Read the model definition and answer for the solid it produces. Units are mm, in the model's axes. A direction names the side the tool comes from. Give positions to 0.01 mm unless a question says otherwise; leave off trailing zeros. Order: outer loops, then holes, each group sorted by start corner. A loop starts at its lowest first (then second) coordinate and runs counter-clockwise, first axis right, second up. Notation, with made-up numbers: (-17.5, -27.5) - (19.5, -27.5) arc R38 cw to (19.5, 10.5) - close; hole circle Ø5 at (14.25, -26). An arc over 180 degrees is marked (long way). Use a Markdown table: item, result. Add a question column.
1. Which of the six approach directions +Z, -Z, +X, -X, +Y, -Y give full straight-line access (tool end or side, diameter ignored) to faces 3 (the flat face through (-1, 7, 0)), 4 (the flat face through (117, 5, -2)), 5 (the flat face through (-1, 3, 30))?
2. A cutting plane is placed at C-C on x = 26.5. Determine the outline of the cut face in (y, z), and give its area (3 significant figures).
3. Consider L1, parallel to X at y = 2.55, z = 90; L2, parallel to X at y = 1, z = 115; L3, parallel to X at y = 4.5, z = 99.5. Determine where each line is inside the solid, lowest interval first.
4. Flat-ended cylindrical pins translate along their axes: P1, Ø6.5, axis at x = -130, z = 115, coming from the -Y side; P2, Ø3, axis at x = -90, y = 1, coming from the -Z side; P3, Ø4.5, axis at x = -129, z = 70, coming from the +Y side; P4, Ø4, axis at x = -92, y = 3.5, coming from the +Z side. Find the tip coordinate at first contact, or state that the pin passes through.
5. A cutting plane is placed at A-A on z = -51.5. Determine the outline of the cut face in (x, y).
6. A cutting plane is placed at B-B on y = 1.25. State how many separate pieces and enclosed holes the cut face has, and give its area (3 significant figures).
7. For a pull along X with two mould halves and no side action, classify faces 1 (the flat face through (-1, 3, -30)), 2 (the flat face through (-118, 5, -2)) as released by +X, released by -X, zero draft, split by the parting line, or undercut.
```python
from build123d import *

# Parameters (mm, degrees)
SKETCH1_W             = 45
SKETCH1_H             = 250
BOSS_EXTRUDE1_DEPTH   = 5
BOSS_EXTRUDE1_2_DEPTH = 5
SKETCH2_W             = 190
SKETCH2_H             = 60
BOSS_EXTRUDE2_DEPTH   = 7
CHAMFER1_SIZE         = 2
FILLET1_R             = 2
SKETCH3_R             = 2
CUT_EXTRUDE1_DEPTH    = 188.749833555
LPATTERN1_COUNT       = 2
LPATTERN1_PITCH       = 240
LPATTERN1_COUNT_DIR2  = 2
LPATTERN1_PITCH_DIR2  = 160
SKETCH4_R             = 4
CUT_EXTRUDE2_DEPTH    = 188.749833555
LPATTERN2_COUNT       = 2
LPATTERN2_PITCH       = 260
LPATTERN2_COUNT_DIR2  = 2
LPATTERN2_PITCH_DIR2  = 230


with BuildPart() as part:
    # Sketch1 → Boss-Extrude1 (new body)
    with BuildSketch(Plane(origin=(0, 0, 0), x_dir=(1, 0, 0), z_dir=(0, 1, 0))):
        with Locations((-117.5, 0)):
            Rectangle(SKETCH1_W, SKETCH1_H)
    extrude(amount=BOSS_EXTRUDE1_DEPTH)



with BuildPart() as body_2:
    # Sketch1 → Boss-Extrude1 2 (new body)
    with BuildSketch(Plane(origin=(0, 0, 0), x_dir=(1, 0, 0), z_dir=(0, 1, 0))):
        with Locations((117.5, 0)):
            Rectangle(SKETCH1_W, SKETCH1_H)
    extrude(amount=BOSS_EXTRUDE1_2_DEPTH)


with BuildPart() as part_1:
    add(part.part)

    add(body_2.part)  # Boss-Extrude2 merges body 2
    # Sketch2 → Boss-Extrude2 (add)
    with BuildSketch(Plane(origin=(0, 0, 0), x_dir=(1, 0, 0), z_dir=(0, 1, 0))):
        Rectangle(SKETCH2_W, SKETCH2_H)
    extrude(amount=BOSS_EXTRUDE2_DEPTH)

    # Chamfer1
    chamfer1_edges = [part_1.edges().sort_by_distance(p)[0] for p in [
        (95, 7, 0),
        (-95, 7, 0),
    ]]
    chamfer(chamfer1_edges, length=CHAMFER1_SIZE - 0.0001)  # a hair under: the kernel refuses the full size

    # Fillet1
    fillet1_edges = [part_1.edges().sort_by_distance(p)[0] for p in [
        (95, 2.5, -125),
        (95, 2.5, 125),
        (140, 2.5, 125),
        (140, 2.5, -125),
        (-95, 2.5, -125),
        (-95, 2.5, 125),
        (-140, 2.5, 125),
        (-140, 2.5, -125),
    ]]
    fillet(fillet1_edges, radius=FILLET1_R)

    # Sketch3 → Cut-Extrude1 (cut, through all)
    with BuildSketch(Plane(origin=(0, 5, 0), x_dir=(1, 0, 0), z_dir=(0, 1, 0))):
        with Locations(Location((-129, 90, 0), (0, 0, 270))):
            Circle(SKETCH3_R)
        with Locations(Location((-111, 90, 0), (0, 0, 270))):
            Circle(SKETCH3_R)
        with Locations(Location((-129, 70, 0), (0, 0, 270))):
            Circle(SKETCH3_R)
        with Locations(Location((-111, 70, 0), (0, 0, 270))):
            Circle(SKETCH3_R)
    cut_extrude1 = extrude(amount=-CUT_EXTRUDE1_DEPTH, mode=Mode.SUBTRACT)

    # LPattern1: Cut-Extrude1 2 × 2
    with Locations(*[(i * LPATTERN1_PITCH, 0, j * LPATTERN1_PITCH_DIR2) for i in range(LPATTERN1_COUNT) for j in range(LPATTERN1_COUNT_DIR2) if (i, j) != (0, 0)]):
        add(cut_extrude1, mode=Mode.SUBTRACT)

    # Sketch4 → Cut-Extrude2 (cut, through all)
    with BuildSketch(Plane(origin=(0, 5, 0), x_dir=(1, 0, 0), z_dir=(0, 1, 0))):
        with Locations(Location((-130, 115, 0), (0, 0, 270))):
            Circle(SKETCH4_R)
    cut_extrude2 = extrude(amount=-CUT_EXTRUDE2_DEPTH, mode=Mode.SUBTRACT)

    # LPattern2: Cut-Extrude2 2 × 2
    with Locations(*[(i * LPATTERN2_PITCH, 0, j * LPATTERN2_PITCH_DIR2) for i in range(LPATTERN2_COUNT) for j in range(LPATTERN2_COUNT_DIR2) if (i, j) != (0, 0)]):
        add(cut_extrude2, mode=Mode.SUBTRACT)


solid = part_1.part
```
Output values:
| question | item | result |
|---|---|---|
| 1 | face 3 | +Z, -Z, +X, -X, +Y |
| 1 | face 4 | +Z, -Z, +X, +Y |
| 1 | face 5 | +Z, +Y, -Y |
| 2 | outline | (0, -30) - (7, -30) - (7, 30) - (0, 30) - close |
| 2 | area | 420 mm² |
| 3 | L1 | -140 to -131, -127 to -113, -109 to -95, 95 to 109, 113 to 127, 131 to 140 |
| 3 | L2 | -140 to -134, -126 to -95, 95 to 126, 134 to 140 |
| 3 | L3 | -140 to -95, 95 to 140 |
| 4 | P1 | through |
| 4 | P2 | z = -30 |
| 4 | P3 | y = 5 |
| 4 | P4 | z = 30 |
| 5 | outline | (-140, 0) - (-95, 0) - (-95, 5) - (-140, 5) - close; (95, 0) - (140, 0) - (140, 5) - (95, 5) - close |
| 6 | separate pieces | 1 |
| 6 | enclosed holes | 20 |
| 6 | area | 33,500 mm² |
| 7 | face 1 | undercut |
| 7 | face 2 | zero draft |
